Geometry: final body of the model. Coordinates: model frame, mm. Face numbers are marked on the shaded views. A direction names the side the tool comes from. Give positions to 0.01 mm unless a question says otherwise; leave off trailing zeros. Write each loop counter-clockwise with the first axis right and the second up, starting at its lowest first coordinate (ties: lowest second). Pieces come first, ordered by that corner, then holes. Notation, with made-up numbers: (78, -20) - (127, -20) arc R18 cw to (127, 0) - close; hole circle Ø10 at (-11, 78.5). An arc over 180 degrees is marked (long way). Use CSV: the item, a comma, the result in double quotes. Start each with the question number.
(1) Section B-B on x = 0. Output: boundary loops of the cut face in (y, z), and give its area (3 significant figures).
(2) Section C-C on y = -4. Output: boundary loops of the cut face in (x, z).
(3) Section D-D on z = 11.5. Output: boundary loops of the cut face in (x, y), and give its area (3 significant figures).
(4) Line query: probe 1 along X at (y, z) = (11.9, 26); probe 2 along Z at (x, y) = (-5, 11.15); probe 3 along Y at (x, z) = (-6.5, -22.5). Output: solid intervals per line, ascending. Write a range as [from, to].
(5) First-contact query: pin 1 Ø4 at (x, z) = (-5, -24.5) entering from +Y; pin 2 Ø10 at (x, y) = (-4.5, -9.5) entering from +Z; pin 3 Ø6.5 at (x, y) = (1, 18) entering from -Z. Flat tips, straight axial feed; report the tip coordinate or a pass-through.
(6) Section A-A on z = -26. Output: boundary loops of the cut face in (x, y), and give its area (4 significant figures).
(7) Reachability of the marked faces 1, 2 and 3 from +Z, -Z, +X, -X, +Y, -Y: full face, straight path, thin tool, end or side. Return the list, or none.
from build123d import *

# Parameters (mm, degrees)
SKETCH_1_W               = 20.5
SKETCH_1_H               = 41
EXTRUDE_1_DEPTH          = 20.5
SKETCH_2_W               = 0.5
SKETCH_2_H               = 0.5
CUT_EXTRUDE_1_DEPTH      = 31.75
SKETCH_3_W               = 0.5
SKETCH_3_H               = 0.5
CUT_EXTRUDE_2_DEPTH      = 31.75
SKETCH_4_W               = 7.5
SKETCH_4_H               = 2.5
EXTRUDE_2_DEPTH          = 10.25
SKETCH_5_R               = 2.25
CUT_EXTRUDE_3_DEPTH      = 45.438328051
FILLET_1_R               = 0.2
FILLET_1_OF_MIRROR_3_R   = 0.2
CUT_EXTRUDE_4_DEPTH      = 37.184423444
CUT_EXTRUDE_4_DEPTH_BACK = 37.184423444
FILLET_2_R               = 0.5
SKETCH_7_R               = 3.5
EXTRUDE_3_DEPTH          = 5


with BuildPart() as part:
    # 스케치1 → 보스-돌출1 (new, symmetric)
    with BuildSketch(Plane(origin=(0, 0, 0), x_dir=(1, 0, 0), z_dir=(0, 1, 0))):
        Rectangle(SKETCH_1_W, SKETCH_1_H)
    extrude(amount=EXTRUDE_1_DEPTH, both=True)

    # 스케치2 → 컷-돌출1 (cut, symmetric)
    with BuildSketch(Plane.XY):
        with Locations((-10.25, 9.7)):
            Rectangle(SKETCH_2_W, SKETCH_2_H)
    cut_extrude_1 = extrude(amount=CUT_EXTRUDE_1_DEPTH, both=True, mode=Mode.SUBTRACT)

    # 대칭 복사1: 컷-돌출1 across plane
    add(cut_extrude_1.mirror(Plane(origin=(0, 0, 0), x_dir=(0, 0, 1), z_dir=(1, 0, 0))), mode=Mode.SUBTRACT)

    # 스케치3 → 컷-돌출2 (cut, symmetric)
    with BuildSketch(Plane(origin=(0, 0, 0), x_dir=(0, 0, -1), z_dir=(1, 0, 0))):
        with Locations((-20.5, 9.7)):
            Rectangle(SKETCH_3_W, SKETCH_3_H)
    cut_extrude_2 = extrude(amount=CUT_EXTRUDE_2_DEPTH, both=True, mode=Mode.SUBTRACT)

    # 대칭 복사2: 컷-돌출2 across plane
    add(cut_extrude_2.mirror(Plane.XY), mode=Mode.SUBTRACT)

    # 스케치4 → 보스-돌출2 (add, symmetric)
    with BuildSketch(Plane(origin=(0, 0, 0), x_dir=(0, 0, -1), z_dir=(1, 0, 0))):
        with Locations((24.25, 11.2)):
            Rectangle(SKETCH_4_W, SKETCH_4_H)
    extrude_2 = extrude(amount=EXTRUDE_2_DEPTH, both=True)

    # 스케치5 → 컷-돌출3 (cut, symmetric)
    with BuildSketch(Plane(origin=(0, 12.45, 0), x_dir=(1, 0, 0), z_dir=(0, 1, 0))):
        with Locations((5, 26)):
            Circle(SKETCH_5_R)
        with Locations((-5, 26)):
            Circle(SKETCH_5_R)
    cut_extrude_3 = extrude(amount=CUT_EXTRUDE_3_DEPTH, both=True, mode=Mode.SUBTRACT)

    # 필렛1
    fillet_1_edges = [part.edges().sort_by_distance(p)[0] for p in [
        (3.969223594, 11.2, -28),
        (6.030776406, 11.2, -28),
        (-6.030776406, 11.2, -28),
        (-3.969223594, 11.2, -28),
    ]]
    fillet(fillet_1_edges, radius=FILLET_1_R)

    # 대칭 복사3: 보스-돌출2, 컷-돌출3 across plane
    add(extrude_2.mirror(Plane.XY))
    add(cut_extrude_3.mirror(Plane.XY), mode=Mode.SUBTRACT)

    # 필렛1 of 대칭 복사3
    fillet_1_of_mirror_3_edges = [part.edges().sort_by_distance(p)[0] for p in [
        (3.969223594, 11.2, 28),
        (6.030776406, 11.2, 28),
        (-6.030776406, 11.2, 28),
        (-3.969223594, 11.2, 28),
    ]]
    fillet(fillet_1_of_mirror_3_edges, radius=FILLET_1_OF_MIRROR_3_R)

    # 스케치6 → 컷-돌출4 (cut, two sides: drawn at the far end of the back side and taken through both)
    with BuildSketch(Plane(origin=(0, 0, 0), x_dir=(0, 0, -1), z_dir=(1, 0, 0)).offset(-CUT_EXTRUDE_4_DEPTH_BACK)):
        Polygon((-20.5, 16), (-20.5, 20.5), (-12.705771366, 20.5), align=None)
    extrude(amount=CUT_EXTRUDE_4_DEPTH + CUT_EXTRUDE_4_DEPTH_BACK, mode=Mode.SUBTRACT)

    # 필렛2
    fillet_2_edges = [part.edges().sort_by_distance(p)[0] for p in [
        (-10.25, -5.525, 20.5),
        (-10.25, -5.525, -20.5),
        (10.25, -5.525, 20.5),
        (10.25, -5.525, -20.5),
        (-10.25, 16.475, -20.5),
        (10.25, 16.475, -20.5),
    ]]
    fillet(fillet_2_edges, radius=FILLET_2_R)

    # 스케치7 → 보스-돌출3 (add)
    with BuildSketch(Plane(origin=(0, 20.5, 0), x_dir=(1, 0, 0), z_dir=(0, 1, 0))):
        with Locations(Location((0, 11, 0), (0, 0, 90))):
            Circle(SKETCH_7_R)
    extrude(amount=EXTRUDE_3_DEPTH)


solid = part.part
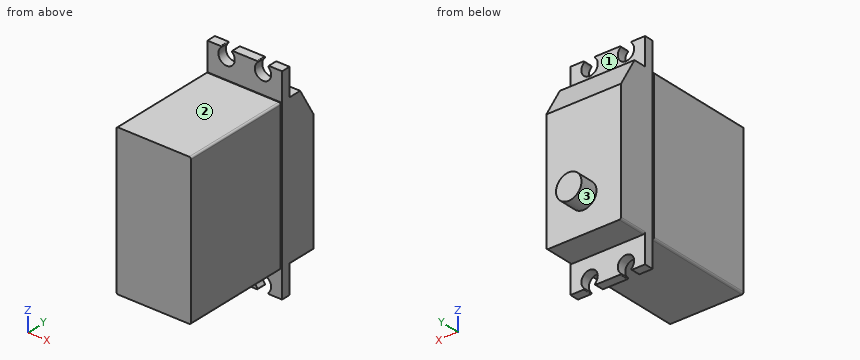
Check values:
1,outline,"(-20.5, -20.5) - (9.45, -20.5) - (9.45, -20.25) - (9.95, -20.25) - (9.95, -28) - (12.45, -28) - (12.45, -20.5) - (20.5, -20.5) - (20.5, -14.5) - (25.5, -14.5) - (25.5, -7.5) - (20.5, -7.5) - (20.5, 12.71) - (16, 20.5) - (12.45, 20.5) - (12.45, 28) - (9.95, 28) - (9.95, 20.25) - (9.45, 20.25) - (9.45, 20.5) - (-20.5, 20.5) - close"
1,area,"1,740 mm²"
2,outline,"(-10.25, -20) arc R0.5 ccw to (-9.75, -20.5) - (9.75, -20.5) arc R0.5 ccw to (10.25, -20) - (10.25, 20) arc R0.5 ccw to (9.75, 20.5) - (-9.75, 20.5) arc R0.5 ccw to (-10.25, 20) - close"
3,outline,"(-10.25, -20.5) - (10.25, -20.5) - (10.25, 9.45) - (10, 9.45) - (10, 9.95) - (10.25, 9.95) - (10.25, 20.5) - (-10.25, 20.5) - (-10.25, 9.95) - (-10, 9.95) - (-10, 9.45) - (-10.25, 9.45) - close"
3,area,"840 mm²"
4,probe 1,"x = [-10.25, -7.25], [-2.75, 2.75], [7.25, 10.25]"
4,probe 2,"z = [-23.75, 23.75]"
4,probe 3,"y = [9.95, 12.45]"
5,pin 1,"stops at y = 12.45"
5,pin 2,"stops at z = 20.5"
5,pin 3,"stops at z = -20.5"
6,outline,"(-10.25, 9.95) - (-7.25, 9.95) - (-7.25, 12.45) - (-10.25, 12.45) - close; (-2.75, 9.95) - (2.75, 9.95) - (2.75, 12.45) - (-2.75, 12.45) - close; (7.25, 9.95) - (10.25, 9.95) - (10.25, 12.45) - (7.25, 12.45) - close"
6,area,"28.75 mm²"
7,face 1,"+Z, +X, -X, +Y"
7,face 2,"+Z, +X, -X, -Y"
7,face 3,"+Y"
